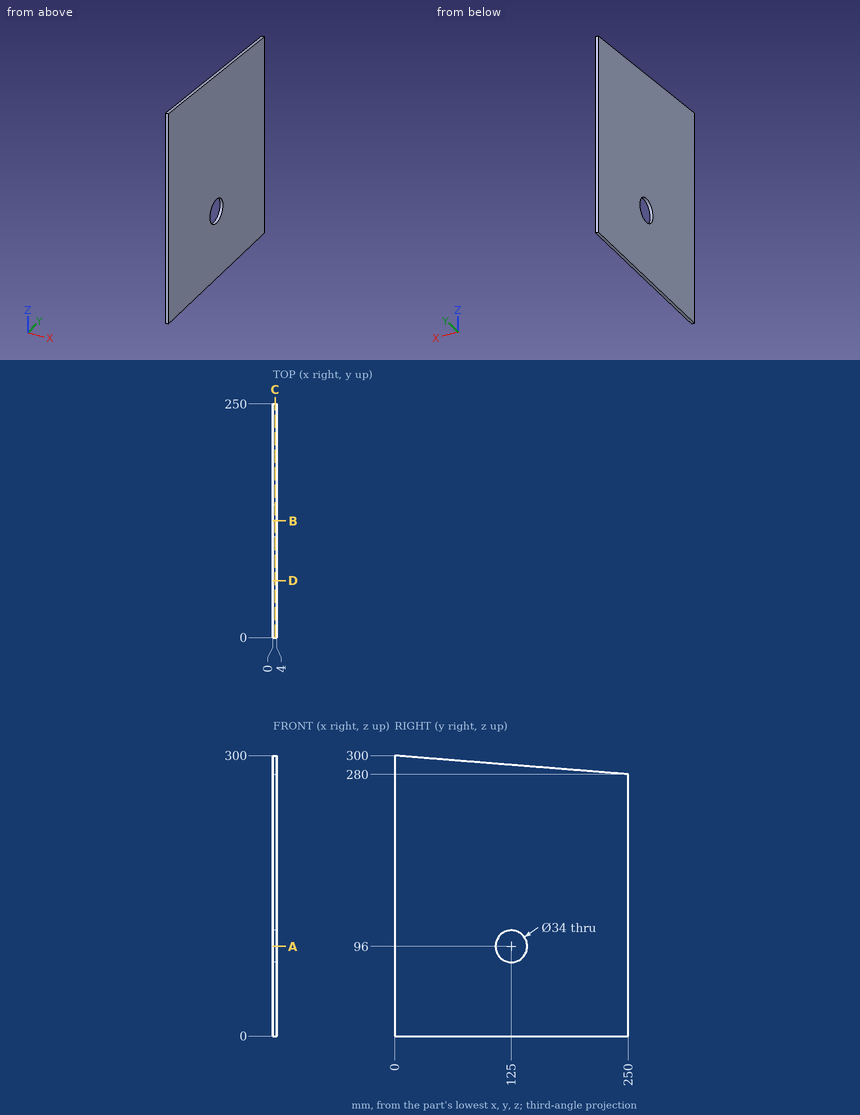
Source: three-view drawing plus pictorial views. Frame: mm from the lowest corner of the part. Coordinates: 2 decimals unless noted, no trailing zeros. Write each loop counter-clockwise with the first axis right and the second up, starting at its lowest first coordinate (ties: lowest second). Pieces come first, ordered by that corner, then holes. Notation, with made-up numbers: (-22, 67) - (-4, 67) arc R10 ccw to (-4, 79) - close; hole circle Ø2 at (88, -4.75). An arc over 180 degrees is marked (long way). Answer as a JSON object with one key per item and string values.
Q1. Section query B-B, the plane y = 125. Output: boundary loops of the cut face in (x, z).
Ans:
{"outline": "(0, 0) - (4, 0) - (4, 79) - (0, 79) - close; (0, 113) - (4, 113) - (4, 290) - (0, 290) - close"}
Q2. Material intervals for line 1 (Z direction, x = 1.9, y = 125); line 2 (Z direction, x = 1.15, y = 130); line 3 (Z direction, x = 1.6, y = 61), sorted ascending. Write a range as [from, to].
Ans:
{"line 1": "z = [0, 79], [113, 290]", "line 2": "z = [0, 79.75], [112.25, 289.6]", "line 3": "z = [0, 295.12]"}
Q3. Section query D-D, the plane y = 61. Output: boundary loops of the cut face in (x, z), plus the area to 3 significant figures.
Ans:
{"outline": "(0, 0) - (4, 0) - (4, 295.12) - (0, 295.12) - close", "area": "1,180 mm2"}
Q4. Section query C-C, the plane x = 2.5. Output: boundary loops of the cut face in (y, z), plus the area to 3 significant figures.
Ans:
{"outline": "(0, 0) - (250, 0) - (250, 280) - (0, 300) - close; hole circle Ø34 at (125, 96)", "area": "71,600 mm2"}
Q5. Section query A-A, the plane z = 96. Output: boundary loops of the cut face in (x, y).
Ans:
{"outline": "(0, 0) - (4, 0) - (4, 108) - (0, 108) - close; (0, 142) - (4, 142) - (4, 250) - (0, 250) - close"}
